Here's how the part is built. I have some questions about the finished solid (model axes, mm). A direction names the side the tool comes from. Give positions to 0.01 mm unless a question says otherwise; leave off trailing zeros. Write each loop counter-clockwise with the first axis right and the second up, starting at its lowest first coordinate (ties: lowest second). Pieces come first, ordered by that corner, then holes. Notation, with made-up numbers: (0, -34.5) - (31, -34.5) arc R20 ccw to (31, -4.5) - close; hole circle Ø11 at (44.25, 14). An arc over 180 degrees is marked (long way). Use a Markdown table: item, result.
```python
from build123d import *

# Parameters (mm, degrees)
CYLINDER066_R     = 1.3
CYLINDER066_DEPTH = 331
CYLINDER070_W     = 105
CYLINDER070_H     = 10
CYLINDER070_ANGLE = 13
CYLINDER065_W     = 115
CYLINDER065_H     = 10
CYLINDER065_ANGLE = 13
FILLET011_R       = 2
CYLINDER068_W     = 105
CYLINDER068_H     = 352
CYLINDER068_ANGLE = 13
CYLINDER067_W     = 115
CYLINDER067_H     = 340
CYLINDER067_ANGLE = 13
BOX103_W          = 320
BOX103_H          = 10
BOX103_DEPTH      = 10
CYLINDER069_W     = 105
CYLINDER069_H     = 10
CYLINDER069_ANGLE = 13
CYLINDER064_W     = 115
CYLINDER064_H     = 10
CYLINDER064_ANGLE = 13
FILLET010_R       = 2


with BuildPart() as cilindro066:
    # Cylinder066 → Cylinder066 (new body)
    with BuildSketch(Plane(origin=(5, 6, 178), x_dir=(0, 0, -1), z_dir=(1, 0, 0))):
        Circle(CYLINDER066_R)
    extrude(amount=CYLINDER066_DEPTH)


with BuildPart() as cilindro070:
    # Cylinder070 → Cylinder070 (revolve)
    with BuildSketch(Plane(origin=(20, 115, 162), x_dir=(0, -1, 0), z_dir=(0, 0, -1))):
        with Locations((52.5, 5)):
            Rectangle(CYLINDER070_W, CYLINDER070_H)
    revolve(axis=Axis((20, 115, 162), (-1, 0, 0)), revolution_arc=CYLINDER070_ANGLE)


with BuildPart() as fillet011:
    # Cylinder065 → Cylinder065 (revolve)
    with BuildSketch(Plane(origin=(20, 115, 162), x_dir=(0, -1, 0), z_dir=(0, 0, -1))):
        with Locations((57.5, 5)):
            Rectangle(CYLINDER065_W, CYLINDER065_H)
    revolve(axis=Axis((20, 115, 162), (-1, 0, 0)), revolution_arc=CYLINDER065_ANGLE)

    # Cut075: cut Cilindro070
    add(cilindro070.part, mode=Mode.SUBTRACT)

    # Fillet011
    fillet011_edges = [fillet011.edges().sort_by_distance(p)[0] for p in [
        (20, 7.819293, 186.744616),
    ]]
    fillet(fillet011_edges, radius=FILLET011_R)


with BuildPart() as cilindro068:
    # Cylinder068 → Cylinder068 (revolve)
    with BuildSketch(Plane(origin=(340, 115, 162), x_dir=(0, -1, 0), z_dir=(0, 0, -1))):
        with Locations((52.5, 176)):
            Rectangle(CYLINDER068_W, CYLINDER068_H)
    revolve(axis=Axis((340, 115, 162), (-1, 0, 0)), revolution_arc=CYLINDER068_ANGLE)


with BuildPart() as cut078:
    # Cylinder067 → Cylinder067 (revolve)
    with BuildSketch(Plane(origin=(340, 115, 162), x_dir=(0, -1, 0), z_dir=(0, 0, -1))):
        with Locations((57.5, 170)):
            Rectangle(CYLINDER067_W, CYLINDER067_H)
    revolve(axis=Axis((340, 115, 162), (-1, 0, 0)), revolution_arc=CYLINDER067_ANGLE)

    # Cut078: cut Cilindro068
    add(cilindro068.part, mode=Mode.SUBTRACT)


with BuildPart() as cut078_1:
    # Cut078 placement: moved
    add(cut078.part.moved(Location((0, -10.1, 0))))


with BuildPart() as cut079:
    # Box103 → Box103 (new body)
    with BuildSketch(Plane(origin=(10, 0, 162), x_dir=(1, 0, 0), z_dir=(0, 0, 1))):
        with Locations((160, 5)):
            Rectangle(BOX103_W, BOX103_H)
    extrude(amount=BOX103_DEPTH)

    # Cut079: cut Cut078
    add(cut078_1.part, mode=Mode.SUBTRACT)


with BuildPart() as cilindro069:
    # Cylinder069 → Cylinder069 (revolve)
    with BuildSketch(Plane(origin=(20, 115, 162), x_dir=(0, -1, 0), z_dir=(0, 0, -1))):
        with Locations((52.5, 5)):
            Rectangle(CYLINDER069_W, CYLINDER069_H)
    revolve(axis=Axis((20, 115, 162), (-1, 0, 0)), revolution_arc=CYLINDER069_ANGLE)


with BuildPart() as cut076:
    # Cylinder064 → Cylinder064 (revolve)
    with BuildSketch(Plane(origin=(20, 115, 162), x_dir=(0, -1, 0), z_dir=(0, 0, -1))):
        with Locations((57.5, 5)):
            Rectangle(CYLINDER064_W, CYLINDER064_H)
    revolve(axis=Axis((20, 115, 162), (-1, 0, 0)), revolution_arc=CYLINDER064_ANGLE)

    # Cut077: cut Cilindro069
    add(cilindro069.part, mode=Mode.SUBTRACT)


with BuildPart() as cut076_1:
    # Cut077 placement: moved
    add(cut076.part.moved(Location((310, 0, 0))))

    # Fillet010
    fillet010_edges = [cut076_1.edges().sort_by_distance(p)[0] for p in [
        (320, 7.819293, 186.744616),
    ]]
    fillet(fillet010_edges, radius=FILLET010_R)

    # Fusion017: union Fillet011, Cut079
    add(fillet011.part)
    add(cut079.part)

    # Cut076: cut Cilindro066
    add(cilindro066.part, mode=Mode.SUBTRACT)


solid = cut076_1.part
```
Item 1: Will these pins go through, and if not, where does the flat tip stop? pin 1 Ø7.5 at (x, y) = (119.5, 5.5) entering from +Z; pin 2 Ø8 at (x, z) = (48, 178) entering from +Y; pin 3 Ø12 at (x, z) = (272, 166.5) entering from +Y.
Values:
| item | result |
|---|---|
| pin 1 | stops at z = 172 |
| pin 2 | passes through |
| pin 3 | stops at y = 10 |
Item 2: If we section it at A-A, the plane x = 207: Write out the boundary of the cut face in (y, z).
Values:
| item | result |
|---|---|
| outline | (0, 162) - (10, 162) - (10, 172) - (0.38, 172) arc R105 ccw to (0, 166.58) - close |
Item 3: For faces 4 (the flat face through (168, 10, 167)), 5 (the flat face through (168, 5, 162)), which set-ups out of +Z, -Z, +X, -X, +Y, -Y let a thin tool reach every point of the face, with its end or its side?
Values:
| item | result |
|---|---|
| face 4 | +Z, -Z, +Y |
| face 5 | -Z, +X, -X, +Y, -Y |
Item 4: Thinking about a two-plate mould opening in X: for faces 1 (the flat face through (13.94, 7.89, 186.73)), 2 (the flat face through (10, 6, 175)), 3 (the flat face through (20, 6.26, 179.44)), which applies, +X half, -X half, draft (parallel to the pull), parting line (faces both ways), or undercut?
Values:
| item | result |
|---|---|
| face 1 | draft |
| face 2 | -X half |
| face 3 | undercut |
Item 5: I need wall thicknesses on line 1 along X through (y, z) = (4, 172.5); line 2 along Z through (x, y) = (300.5, 4.75); line 3 along Y through (x, z) = (326.75, 178). Which ranges of each line are inside material? Lowest first, please. Write a range as [from, to].
Values:
| item | result |
|---|---|
| line 1 | x = [10, 20], [320, 330] |
| line 2 | z = [162, 172] |
| line 3 | y = [1.12, 4.7], [7.3, 11.23] |
